For this review, take the finished solid that the model builds, in its own axes (mm). Face numbers are marked on the shaded views. A direction names the side the tool comes from. Round coordinates to 2 decimals unless told otherwise and drop trailing zeros. Write each loop counter-clockwise with the first axis right and the second up, starting at its lowest first coordinate (ties: lowest second). Pieces come first, ordered by that corner, then holes. Notation, with made-up numbers: M -30.5,29.25 L -3.5,29.25 A17 cw -3.5,39.25 Z; hole C -11,75 d5. An arc over 180 degrees is marked long. Use one line per item in the form item = value. Start each with the question number.
Item 1: Add section A-A (z = -15). State the section outline as (x, y) points.
Item 2: Add section C-C (y = 67). State the section outline as (x, z) points, and give its area (3 significant figures).
Item 3: For line 1 (X direction, y = 0.85, z = -15); line 2 (X direction, y = 4.55, z = -15); line 3 (Z direction, x = 7, y = 39.5), list the stretches that pass through material, from the lowest coordinate up. Write a range as [from, to].
Item 4: For P1, Ø6.5, axis at x = -25, z = -15, coming from the +Y side; P2, Ø3, axis at x = 46.5, z = 7, coming from the +Y side, all flat-tipped, find the tip position at first contact; note any pin that passes through.
Item 5: For the marked faces 1 and 2, list the 3-axis set-ups (+Z, -Z, +X, -X, +Y, -Y) from which the entire face can be reached by the end or side of a thin tool; tool diameter is ignored.
Item 6: Add section B-B (x = 25). State the section outline as (y, z) points, and give its area (3 significant figures).
Item 7: Add section D-D (x = 60). State the section outline as (y, z) points.
from build123d import *

# Parameters (mm, degrees)
SKETCH2_W           = 150
SKETCH2_H           = 60
BOSS_EXTRUDE2_DEPTH = 5
SKETCH3_W           = 150
SKETCH3_H           = 10
BOSS_EXTRUDE3_DEPTH = 100
SKETCH4_R           = 3.5
CUT_EXTRUDE1_DEPTH  = 129.549601322
SKETCH6_R           = 5
CUT_EXTRUDE2_DEPTH  = 1


with BuildPart() as part:
    # Sketch2 → Boss-Extrude2 (new body)
    with BuildSketch(Plane(origin=(0, 0, 0), x_dir=(1, 0, 0), z_dir=(0, 1, 0))):
        Rectangle(SKETCH2_W, SKETCH2_H)
    extrude(amount=BOSS_EXTRUDE2_DEPTH)

    # Sketch3 → Boss-Extrude3 (add)
    with BuildSketch(Plane(origin=(0, 5, 0), x_dir=(1, 0, 0), z_dir=(0, 1, 0))):
        with Locations((0, -25)):
            Rectangle(SKETCH3_W, SKETCH3_H)
    extrude(amount=BOSS_EXTRUDE3_DEPTH)

    # Sketch4 → Cut-Extrude1 (cut, through all)
    with BuildSketch(Plane(origin=(0, 5, 0), x_dir=(1, 0, 0), z_dir=(0, 1, 0))):
        with Locations(Location((-25, 15, 0), (0, 0, 270))):
            Circle(SKETCH4_R)
        with Locations(Location((25, 15, 0), (0, 0, 270))):
            Circle(SKETCH4_R)
    extrude(amount=-CUT_EXTRUDE1_DEPTH, mode=Mode.SUBTRACT)

    # Sketch6 → Cut-Extrude2 (cut)
    with BuildSketch(Plane(origin=(0, 5, 0), x_dir=(1, 0, 0), z_dir=(0, 1, 0))):
        with Locations(Location((-25, 15, 0), (0, 0, 270))):
            Circle(SKETCH6_R)
        with Locations(Location((25, 15, 0), (0, 0, 270))):
            Circle(SKETCH6_R)
    extrude(amount=-CUT_EXTRUDE2_DEPTH, mode=Mode.SUBTRACT)


solid = part.part
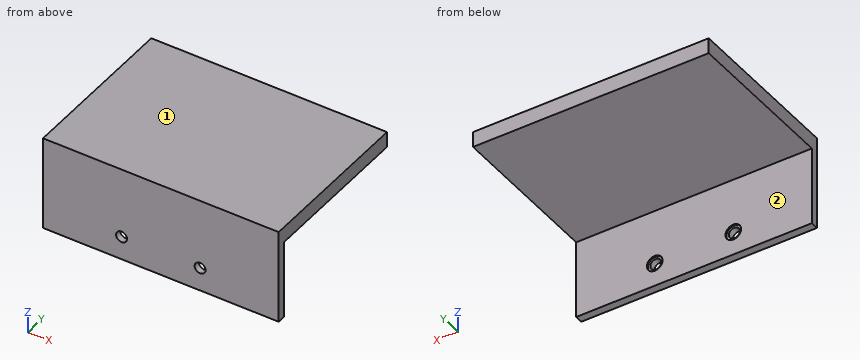
Calculated:
q1.outline = M -75,0 L -28.5,0 L -28.5,4 L -30,4 L -30,5 L -75,5 Z; M -21.5,0 L 21.5,0 L 21.5,4 L 20,4 L 20,5 L -20,5 L -20,4 L -21.5,4 Z; M 28.5,0 L 75,0 L 75,5 L 30,5 L 30,4 L 28.5,4 Z
q2.outline = M -75,20 L 75,20 L 75,30 L -75,30 Z
q2.area = 1,500 mm^2
q3.line_1 = [-75, -28.5], [-21.5, 21.5], [28.5, 75]
q3.line_2 = [-75, -30], [-20, 20], [30, 75]
q3.line_3 = [20, 30]
q4.P1 = through
q4.P2 = 5
q5.face_1 = +Z, +X, -X, +Y, -Y
q5.face_2 = -Z, +X, -X, +Y
q6.outline = M 0,-30 L 5,-30 L 5,-20 L 4,-20 L 4,-18.5 L 0,-18.5 Z; M 0,-11.5 L 4,-11.5 L 4,-10 L 5,-10 L 5,20 L 105,20 L 105,30 L 0,30 Z
q6.area = 1,260 mm^2
q7.outline = M 0,-30 L 5,-30 L 5,20 L 105,20 L 105,30 L 0,30 Z
